Part print with two shaded views. Sizes in mm from the minimum x, y, z corner. A direction names the side the tool comes from. Coordinates: 2 decimals unless noted, no trailing zeros. Write each loop counter-clockwise with the first axis right and the second up, starting at its lowest first coordinate (ties: lowest second). Pieces come first, ordered by that corner, then holes. Notation, with made-up numbers: (49.25, -28) -> (58.25, -28) arc R24 ccw to (58.25, 5) -> close; hole circle Ø3 at (33.5, 25). An arc over 180 degrees is marked (long way). Write item = value, one per line. Start each with the question number.
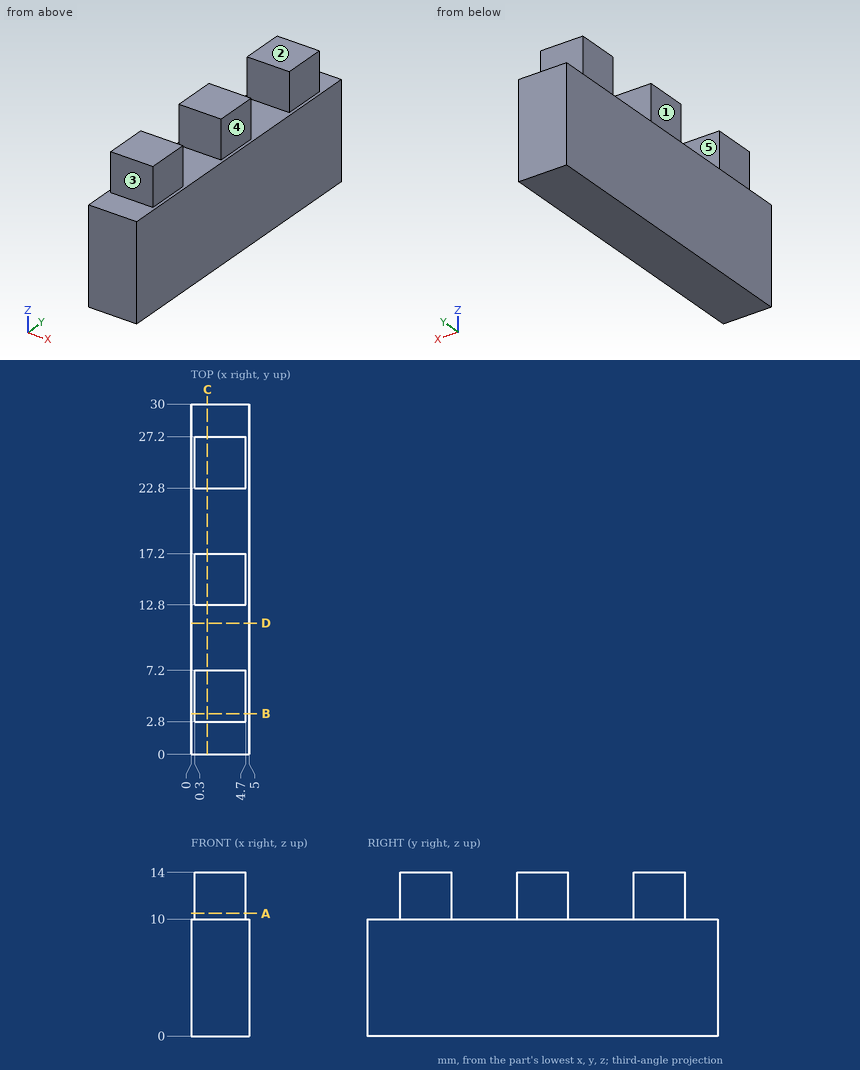
(1) Drop flat-ended pins along their axis: pin 1 Ø1.5 at (x, y) = (3, 16) entering from -Z; pin 2 Ø2 at (y, z) = (14.5, 11.5) entering from +X; pin 3 Ø1.2 at (y, z) = (15, 12) entering from -X; pin 4 Ø1.2 at (x, z) = (3, 11.5) entering from +Y. Give the stop position or say it passes through.
(2) Saw through at C-C (x = 1.4). Give the cut face in (y, z).
(3) 3-axis set-ups, long thin cutter, end or side, ignore diameter. For the marked faces 1, 2, 3, 4 and 5: which of +Z, -Z, +X, -X, +Y, -Y reach the whole face in a straight line?
(4) Drill centre lines: line 1 along X through (y, z) = (23.5, 12.5); line 2 along Z through (x, y) = (0.8, 20.5). Where is each one in solid material? Low to high.
(5) Saw through at A-A (z = 10.5). Give the cut face in (x, y), then the cut area to 3 significant figures.
(6) Saw through at B-B (y = 3.5). Give the cut face in (x, z).
(7) Saw through at D-D (y = 11.25). Give the cut face in (x, z), then the cut area to 3 significant figures.
Returned:
q1.pin_1 = 0
q1.pin_2 = 4.7
q1.pin_3 = 0.3
q1.pin_4 = 27.2
q2.outline = (0, 0) -> (30, 0) -> (30, 10) -> (27.2, 10) -> (27.2, 14) -> (22.8, 14) -> (22.8, 10) -> (17.2, 10) -> (17.2, 14) -> (12.8, 14) -> (12.8, 10) -> (7.2, 10) -> (7.2, 14) -> (2.8, 14) -> (2.8, 10) -> (0, 10) -> close
q3.face_1 = +Z, -X, +Y, -Y
q3.face_2 = +Z, +X, -X, +Y, -Y
q3.face_3 = +Z, +X, -X, -Y
q3.face_4 = +Z, +X, +Y, -Y
q3.face_5 = +Z, +X, -X
q4.line_1 = 0.3 to 4.7
q4.line_2 = 0 to 10
q5.outline = (0.3, 2.8) -> (4.7, 2.8) -> (4.7, 7.2) -> (0.3, 7.2) -> close; (0.3, 12.8) -> (4.7, 12.8) -> (4.7, 17.2) -> (0.3, 17.2) -> close; (0.3, 22.8) -> (4.7, 22.8) -> (4.7, 27.2) -> (0.3, 27.2) -> close
q5.area = 58.1 mm2
q6.outline = (0, 0) -> (5, 0) -> (5, 10) -> (4.7, 10) -> (4.7, 14) -> (0.3, 14) -> (0.3, 10) -> (0, 10) -> close
q7.outline = (0, 0) -> (5, 0) -> (5, 10) -> (0, 10) -> close
q7.area = 50.0 mm2
